Design review of the part built by this model. Coordinates are the model's own, in mm. Face numbers are marked on the shaded views. A direction names the side the tool comes from. Round coordinates to 2 decimals unless told otherwise and drop trailing zeros. Order: outer loops, then holes, each group sorted by start corner. A loop starts at its lowest first (then second) coordinate and runs counter-clockwise, first axis right, second up.
from build123d import *

# Parameters (mm, degrees)
SKETCH_1_W          = 83.5
SKETCH_1_H          = 28
EXTRUDE_1_DEPTH     = 5
SKETCH_2_R          = 5.5
EXTRUDE_2_DEPTH     = 5
EXTRUDE_START       = -5
SKETCH_3_R          = 5.5
EXTRUDE_3_DEPTH     = 5
SKETCH_4_R          = 2.6
CUT_EXTRUDE_2_DEPTH = 5
EXTRUDE_4_DEPTH     = 2.5


with BuildPart() as part:
    # 草图1 → 凸台-拉伸1 (new body)
    with BuildSketch(Plane.XY):
        Rectangle(SKETCH_1_W, SKETCH_1_H)
    extrude(amount=EXTRUDE_1_DEPTH)

    # 草图2 → 凸台-拉伸2 (add)
    with BuildSketch(Plane.ZY.offset(41.75)):
        with BuildLine():
            Line((5, 14), (5, -14))
            Line((5, -14), (43.622842344, -20.810249177))
            ThreePointArc((43.622842344, -20.810249177), (52.5727616, -15.355809237), (48.296475179, -5.786831015))
            Line((48.296475179, -5.786831015), (5, 14))
        make_face()
        with Locations(Location((45, -13, 0), (0, 0, 270))):
            Circle(SKETCH_2_R, mode=Mode.SUBTRACT)
    extrude(amount=-EXTRUDE_2_DEPTH)

    # 草图3 → 凸台-拉伸3 (add)
    with BuildSketch(Plane(origin=(41.75, 0, 0), x_dir=(0, 0, -1), z_dir=(1, 0, 0)).offset(EXTRUDE_START)):
        with BuildLine():
            Line((-5, 14), (-48.296475179, -5.786831015))
            ThreePointArc((-48.296475179, -5.786831015), (-52.5727616, -15.355809237), (-43.622842344, -20.810249177))
            Line((-43.622842344, -20.810249177), (-5, -14))
            Line((-5, -14), (-5, 14))
        make_face()
        with Locations(Location((-45, -13, 0), (0, 0, 270))):
            Circle(SKETCH_3_R, mode=Mode.SUBTRACT)
    extrude(amount=EXTRUDE_3_DEPTH)

    # 草图4 → 切除-拉伸2 (cut)
    with BuildSketch(Plane.XY.offset(5)):
        with Locations((-25, 10)):
            Circle(SKETCH_4_R)
        with Locations((25, 10)):
            Circle(SKETCH_4_R)
        with Locations((25, -10)):
            Circle(SKETCH_4_R)
        with Locations((-25, -10)):
            Circle(SKETCH_4_R)
    extrude(amount=-CUT_EXTRUDE_2_DEPTH, mode=Mode.SUBTRACT)

    # 草图5 → 凸台-拉伸4 (add, symmetric)
    with BuildSketch(Plane(origin=(0, 0, 0), x_dir=(1, 0, 0), z_dir=(0, 1, 0))):
        Polygon((-36.75, -5), (-21.75, -5), (-36.75, -25), align=None)
        Polygon((36.75, -5), (36.75, -25.085459481), (21.75, -5), align=None)
    extrude(amount=EXTRUDE_4_DEPTH, both=True)


solid = part.part
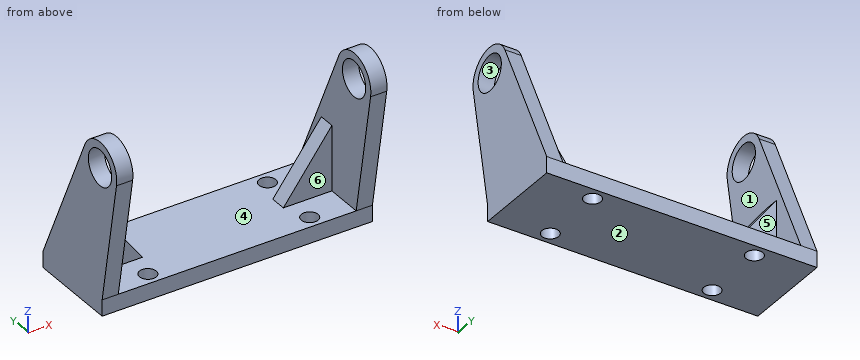
1) Take a section at D-D on x = -25. Give the boundary of the cut face in (y, z).
Results:
outline: (-14, 0) - (-12.6, 0) - (-12.6, 5) - (-14, 5) - close; (-7.4, 0) - (7.4, 0) - (7.4, 5) - (2.5, 5) - (2.5, 9.33) - (-2.5, 9.33) - (-2.5, 5) - (-7.4, 5) - close; (12.6, 0) - (14, 0) - (14, 5) - (12.6, 5) - close
2) Take a section at A-A on y = -10. Give the boundary of the cut face in (x, z).
Results:
outline: (-41.75, 0) - (-27.6, 0) - (-27.6, 5) - (-36.75, 5) - (-36.75, 40.39) - (-41.75, 40.39) - close; (-41.75, 49.61) - (-36.75, 49.61) - (-36.75, 52.34) - (-41.75, 52.34) - close; (-22.4, 0) - (22.4, 0) - (22.4, 5) - (-22.4, 5) - close; (27.6, 0) - (41.75, 0) - (41.75, 40.39) - (36.75, 40.39) - (36.75, 5) - (27.6, 5) - close; (36.75, 49.61) - (41.75, 49.61) - (41.75, 52.34) - (36.75, 52.34) - close
3) The part is to be moulded in two halves that separate along Z. For the marked faces 1, 2 and 3, say which applies: released by +Z, released by -Z, zero draft, split by the parting line, or undercut.
Results:
face 1: zero draft
face 2: released by -Z
face 3: undercut
4) Take a section at B-B on z = 22.5. Give the boundary of the cut face in (x, y) (3 decimals).
Results:
outline: (-41.75, -17.086) - (-36.75, -17.086) - (-36.75, -2.5) - (-34.875, -2.5) - (-34.875, 2.5) - (-36.75, 2.5) - (-36.75, 6.002) - (-41.75, 6.002) - close; (34.819, -2.5) - (36.75, -2.5) - (36.75, -17.086) - (41.75, -17.086) - (41.75, 6.002) - (36.75, 6.002) - (36.75, 2.5) - (34.819, 2.5) - close
5) Clearance check with flat-ended pins moving along their axes: P1, Ø8, axis at x = 20.5, y = -16.5, coming from the +Z side; P2, Ø1.5, axis at x = -17.5, z = 3.5, coming from the -Y side; P3, Ø6.5, axis at y = -13, z = 45, coming from the +X side; P4, Ø1, axis at x = -32, y = 0, coming from the -Z side. State where each tip first meets the part, or that it passes through.
Results:
P1: stops at z = 5
P2: stops at y = -14
P3: passes through
P4: stops at z = 0
6) To check wall thickness, follow line 1 along X through (y, z) = (3, 17); line 2 along Y through (x, z) = (25, 3); line 3 along Y through (x, z) = (28.5, 8). State the ranges of each line that lie inside material, in increasing order.
Results:
line 1: x = -41.75 to -36.75, 36.75 to 41.75
line 2: y = -14 to -12.6, -7.4 to 7.4, 12.6 to 14
line 3: y = -2.5 to 2.5
7) Take a section at C-C on z = 45. Give the boundary of the cut face in (x, y), plus the area to 3 significant figures.
Results:
outline: (-41.75, -20.93) - (-36.75, -20.93) - (-36.75, -18.5) - (-41.75, -18.5) - close; (-41.75, -7.5) - (-36.75, -7.5) - (-36.75, -4.28) - (-41.75, -4.28) - close; (36.75, -20.93) - (41.75, -20.93) - (41.75, -18.5) - (36.75, -18.5) - close; (36.75, -7.5) - (41.75, -7.5) - (41.75, -4.28) - (36.75, -4.28) - close
area: 56.5 mm2
8) For the marked faces 4, 5 and 6, list the 3-axis set-ups (+Z, -Z, +X, -X, +Y, -Y) from which the entire face can be reached by the end or side of a thin tool; tool diameter is ignored.
Results:
face 4: +Z
face 5: +Z, +Y
face 6: +Z, -Y
